from build123d import *

# Parameters (mm, degrees)
SKETCH1_W           = 55
SKETCH1_H           = 57
BOSS_EXTRUDE1_DEPTH = 45.5
SKETCH2_W           = 55
SKETCH2_H           = 38
CUT_EXTRUDE1_DEPTH  = 35.5
SKETCH3_R           = 1.9
CUT_EXTRUDE2_DEPTH  = 10
SKETCH4_R           = 1.9
CUT_EXTRUDE3_DEPTH  = 20


with BuildPart() as part:
    # Sketch1 → Boss-Extrude1 (new body)
    with BuildSketch(Plane.XY):
        Rectangle(SKETCH1_W, SKETCH1_H)
    extrude(amount=BOSS_EXTRUDE1_DEPTH)

    # Sketch2 → Cut-Extrude1 (cut)
    with BuildSketch(Plane.XY.offset(45.5)):
        Rectangle(SKETCH2_W, SKETCH2_H)
    extrude(amount=-CUT_EXTRUDE1_DEPTH, mode=Mode.SUBTRACT)

    # Sketch3 → Cut-Extrude2 (cut)
    with BuildSketch(Plane(origin=(0, 0, 0), x_dir=(-1, 0, 0), z_dir=(0, 0, -1))):
        with Locations((-13.75, 0)):
            Circle(SKETCH3_R)
        with Locations((13.75, 0)):
            Circle(SKETCH3_R)
    extrude(amount=-CUT_EXTRUDE2_DEPTH, mode=Mode.SUBTRACT)

    # Sketch4 → Cut-Extrude3 (cut)
    with BuildSketch(Plane.XY.offset(45.5)):
        with Locations((-12.5, 23.75)):
            Circle(SKETCH4_R)
        with Locations((12.5, 23.75)):
            Circle(SKETCH4_R)
        with Locations((-12.5, -23.75)):
            Circle(SKETCH4_R)
        with Locations((12.5, -23.75)):
            Circle(SKETCH4_R)
    extrude(amount=-CUT_EXTRUDE3_DEPTH, mode=Mode.SUBTRACT)


solid = part.part
Could you check a few things on this model? Use its own coordinates, in mm. A direction names the side the tool comes from. Round coordinates to 2 decimals unless told otherwise and drop trailing zeros. Write each loop counter-clockwise with the first axis right and the second up, starting at its lowest first coordinate (ties: lowest second). Pieces come first, ordered by that corner, then holes. Notation, with made-up numbers: (88.5, -33.5) - (145.5, -33.5) arc R8 ccw to (145.5, -24.5) - close; hole circle Ø6 at (-18, 64.5). An arc over 180 degrees is marked (long way). Use a Markdown table: item, result.
Q1. Thinking about a two-plate mould opening in Y: for faces 1 (the flat face through (0, 28.5, 22)), 2 (the flat face through (27.5, -7, 7)), 3 (the flat face through (0, -28.5, 22)), 4 (the cylindrical face through (15.65, 0.08, 4.93)), which applies, released by +Y, released by -Y, zero draft, split by the parting line, or undercut?
Output values:
| item | result |
|---|---|
| face 1 | released by +Y |
| face 2 | zero draft |
| face 3 | released by -Y |
| face 4 | undercut |
Q2. For faces 5 (the cylindrical face through (-11.85, 0.08, 4.93)), 6 (the flat face through (0, -19, 28)), 7 (the cylindrical face through (12.253, -21.866, 35.64)), which set-ups out of +Z, -Z, +X, -X, +Y, -Y let a thin tool reach every point of the face, with its end or its side?
Output values:
| item | result |
|---|---|
| face 5 | +Z, -Z |
| face 6 | +Z, +X, -X |
| face 7 | +Z |
Q3. For pin 1 (1.5 mm diameter, centred on x = -4, y = -2.5, fed in from +Z); pin 2 (3 mm diameter, centred on x = -12.5, y = -23.75, fed in from +Z); pin 3 (6 mm diameter, centred on x = 12.5, y = 23.75, fed in from -Z); pin 4 (3.5 mm diameter, centred on x = 13.75, y = 0, fed in from +Z), each with a flat end and sliding along its axis, tell me the tip position at first contact or that it passes through.
Output values:
| item | result |
|---|---|
| pin 1 | z = 10 |
| pin 2 | z = 25.5 |
| pin 3 | z = 0 |
| pin 4 | through |
Q4. I want a section at C-C (z = 28). List the corners of the cut face in (x, y) for me, plus the area to 4 significant figures.
Output values:
| item | result |
|---|---|
| outline | (-27.5, -28.5) - (27.5, -28.5) - (27.5, -19) - (-27.5, -19) - close; (-27.5, 19) - (27.5, 19) - (27.5, 28.5) - (-27.5, 28.5) - close; hole circle Ø3.8 at (-12.5, -23.75); hole circle Ø3.8 at (-12.5, 23.75); hole circle Ø3.8 at (12.5, -23.75); hole circle Ø3.8 at (12.5, 23.75) |
| area | 1,000 mm2 |
Q5. Please list where these lines run through material, in increasing order: L1, parallel to Y at x = -12.5, z = 32.5; L2, parallel to Y at x = -16.5, z = 17; L3, parallel to X at y = -23, z = 37.
Output values:
| item | result |
|---|---|
| L1 | -28.5 to -25.65, -21.85 to -19, 19 to 21.85, 25.65 to 28.5 |
| L2 | -28.5 to -19, 19 to 28.5 |
| L3 | -27.5 to -14.25, -10.75 to 10.75, 14.25 to 27.5 |
Q6. I want a section at D-D (x = 9). List the corners of the cut face in (y, z) for me, plus the area to 3 significant figures.
Output values:
| item | result |
|---|---|
| outline | (-28.5, 0) - (28.5, 0) - (28.5, 45.5) - (19, 45.5) - (19, 10) - (-19, 10) - (-19, 45.5) - (-28.5, 45.5) - close |
| area | 1,240 mm2 |
Q7. I want a section at B-B (z = 21). List the corners of the cut face in (x, y) for me.
Output values:
| item | result |
|---|---|
| outline | (-27.5, -28.5) - (27.5, -28.5) - (27.5, -19) - (-27.5, -19) - close; (-27.5, 19) - (27.5, 19) - (27.5, 28.5) - (-27.5, 28.5) - close |
Q8. I want a section at A-A (y = 0). List the corners of the cut face in (x, z) for me, plus the area to 3 significant figures.
Output values:
| item | result |
|---|---|
| outline | (-27.5, 0) - (-15.65, 0) - (-15.65, 10) - (-27.5, 10) - close; (-11.85, 0) - (11.85, 0) - (11.85, 10) - (-11.85, 10) - close; (15.65, 0) - (27.5, 0) - (27.5, 10) - (15.65, 10) - close |
| area | 474 mm2 |
